The listing builds one solid part. Answer for the finished solid, in the listing's coordinates (mm). Give positions to 0.01 mm unless a question says otherwise; leave off trailing zeros. Order: outer loops, then holes, each group sorted by start corner. A loop starts at its lowest first (then second) coordinate and runs counter-clockwise, first axis right, second up. Notation, with made-up numbers: M -4,26 L 6,26 A24 cw 6,65 Z; hole C -38.5,46 d8. An arc over 180 degrees is marked long. Answer as a JSON object with one key per item and string values. Group by question number.
```python
from build123d import *

# Parameters (mm, degrees)
CROQUIS1_W              = 620
CROQUIS1_H              = 320
CROQUIS1_W_2            = 190
CROQUIS1_H_2            = 290
SALIENTE_EXTRUIR1_DEPTH = 10
CROQUIS2_W              = 600
CROQUIS2_H              = 300
CORTAR_EXTRUIR1_DEPTH   = 3


with BuildPart() as part:
    # Croquis1 → Saliente-Extruir1 (new body)
    with BuildSketch(Plane.XY):
        with Locations((300, 150)):
            Rectangle(CROQUIS1_W, CROQUIS1_H)
        with Locations((100, 150)):
            Rectangle(CROQUIS1_W_2, CROQUIS1_H_2, mode=Mode.SUBTRACT)
        with Locations((500, 150)):
            Rectangle(CROQUIS1_W_2, CROQUIS1_H_2, mode=Mode.SUBTRACT)
        with Locations((300, 150)):
            Rectangle(CROQUIS1_W_2, CROQUIS1_H_2, mode=Mode.SUBTRACT)
    extrude(amount=SALIENTE_EXTRUIR1_DEPTH)

    # Croquis2 → Cortar-Extruir1 (cut)
    with BuildSketch(Plane(origin=(0, 0, 0), x_dir=(-1, 0, 0), z_dir=(0, 0, -1))):
        with Locations((-300, 150)):
            Rectangle(CROQUIS2_W, CROQUIS2_H)
    extrude(amount=-CORTAR_EXTRUIR1_DEPTH, mode=Mode.SUBTRACT)


solid = part.part
```
Item 1: Section C-C (z = 7.5) is taken. Determine the outline of the cut face in (x, y), and give its area (3 significant figures).
Item 2: Consider probe 1 along X at (y, z) = (135, 4.75); probe 2 along Y at (x, z) = (554.5, 0.5); probe 3 along Y at (x, z) = (22.5, 5.5). Determine where each line is inside the solid, lowest interval first. Write a range as from..to.
Item 3: Section A-A (y = 196) is taken. Determine the outline of the cut face in (x, z), and give its area (3 significant figures).
Item 4: Section B-B (x = 161) is taken. Determine the outline of the cut face in (y, z), and give its area (3 significant figures).
Values found:
{
 "1": {"outline": "M -10,-10 L 610,-10 L 610,310 L -10,310 Z; hole M 5,5 L 195,5 L 195,295 L 5,295 Z; hole M 205,5 L 395,5 L 395,295 L 205,295 Z; hole M 405,5 L 595,5 L 595,295 L 405,295 Z", "area": "33,100 mm^2"},
 "2": {"probe 1": "x = -10..5, 195..205, 395..405, 595..610", "probe 2": "y = -10..0, 300..310", "probe 3": "y = -10..5, 295..310"},
 "3": {"outline": "M -10,0 L 0,0 L 0,3 L 5,3 L 5,10 L -10,10 Z; M 195,3 L 205,3 L 205,10 L 195,10 Z; M 395,3 L 405,3 L 405,10 L 395,10 Z; M 595,3 L 600,3 L 600,0 L 610,0 L 610,10 L 595,10 Z", "area": "410 mm^2"},
 "4": {"outline": "M -10,0 L 0,0 L 0,3 L 5,3 L 5,10 L -10,10 Z; M 295,3 L 300,3 L 300,0 L 310,0 L 310,10 L 295,10 Z", "area": "270 mm^2"}
}
